from build123d import *

# Parameters (mm, degrees)
SKETCH2_R          = 1.905
CUT_EXTRUDE1_DEPTH = 2.54


with BuildPart() as part:
    # Sketch1 → Revolve1 (revolve)
    with BuildSketch(Plane.XY, mode=Mode.PRIVATE) as revolve1_sk:
        with BuildLine():
            Line((0, 0), (0.79375, 0))
            Line((0.79375, 0), (0.79375, 19.05))
            ThreePointArc((0.79375, 19.05), (0, 19.84375), (-0.79375, 19.05))
            Line((-0.79375, 19.05), (-0.79375, 0))
            Line((-0.79375, 0), (0, 0))
        make_face()
    revolve(revolve1_sk.sketch.rotate(Axis((0, 0, 0), (-1, 0, 0)), 90), axis=Axis((0, 0, 0), (-1, 0, 0)))

    # Sketch2 → Cut-Extrude1 (cut)
    with BuildSketch(Plane(origin=(0.79375, 0, 0), x_dir=(0, 0, -1), z_dir=(1, 0, 0))):
        with BuildLine():
            Line((-4.760272123, 13.32409501), (0, 4.036897437))
            Line((0, 4.036897437), (0, 14.472999652))
            ThreePointArc((0, 14.472999652), (-2.448477719, 14.181708244), (-4.760272123, 13.32409501))
        make_face()
        with BuildLine():
            Line((0, 14.472999652), (0, 4.036897437))
            Line((0, 4.036897437), (4.760272123, 13.32409501))
            ThreePointArc((4.760272123, 13.32409501), (2.448477719, 14.181708244), (0, 14.472999652))
        make_face()
        with BuildLine():
            ThreePointArc((11.200962399, 8.644659614), (13.764640629, 4.472402852), (14.142972367, -0.409916029))
            Line((14.142972367, -0.409916029), (3.839317613, 1.247469913))
            Line((3.839317613, 1.247469913), (11.200962399, 8.644659614))
        make_face()
        with BuildLine():
            ThreePointArc((11.682847592, -7.981401547), (8.507015752, -11.708902678), (3.980565502, -13.577437048))
            Line((3.980565502, -13.577437048), (2.372828779, -3.265918631))
            Line((2.372828779, -3.265918631), (11.682847592, -7.981401547))
        make_face()
        with BuildLine():
            ThreePointArc((-3.980565502, -13.577437048), (-8.507015752, -11.708902678), (-11.682847592, -7.981401547))
            Line((-11.682847592, -7.981401547), (-2.372828779, -3.265918631))
            Line((-2.372828779, -3.265918631), (-3.980565502, -13.577437048))
        make_face()
        with BuildLine():
            Line((-3.839317613, 1.247469913), (-11.200962399, 8.644659614))
            ThreePointArc((-11.200962399, 8.644659614), (-13.764640629, 4.472402852), (-14.142972367, -0.409916029))
            Line((-14.142972367, -0.409916029), (-3.839317613, 1.247469913))
        make_face()
        Circle(SKETCH2_R)
    extrude(amount=-CUT_EXTRUDE1_DEPTH, mode=Mode.SUBTRACT)


solid = part.part
Can you work these out from the model? Positions are in its coordinate system, mm. A direction names the side the tool comes from. Round coordinates to 2 decimals unless told otherwise and drop trailing zeros. Write each loop counter-clockwise with the first axis right and the second up, starting at its lowest first coordinate (ties: lowest second). Pieces come first, ordered by that corner, then holes. Notation, with made-up numbers: M 67.5,8.5 L 101.5,8.5 A24 cw 101.5,38.5 Z; hole C 10,-37 d4. An arc over 180 degrees is marked long. Use a Markdown table: item, result.
Item 1: I want a section at A-A (x = 0). List the corners of the cut face in (y, z) for me (1 decimal).
Found:
| item | result |
|---|---|
| outline | C 0,0 d39.7; hole M -13.6,-4 A10.4 ccw -8,-11.7 L -3.3,-2.4 Z; hole M -13.6,4 L -3.3,2.4 L -8,11.7 A10.4 ccw Z; hole C 0,0 d3.8; hole M -0.4,-14.1 A10.4 ccw 8.6,-11.2 L 1.2,-3.8 Z; hole M -0.4,14.1 L 1.2,3.8 L 8.6,11.2 A10.4 ccw Z; hole M 4,0 L 13.3,-4.8 A10.4 ccw 13.3,4.8 Z |
Item 2: I want a section at B-B (y = 5). State how many separate pieces and enclosed holes the cut face has, and give its area (3 significant figures).
Found:
| item | result |
|---|---|
| separate pieces | 4 |
| enclosed holes | 0 |
| area | 39.8 mm2 |
Item 3: We'd pull the mould along Z, two halves only. Please class faces 1 (the face through (0.794, 4, -0.3)), 2 (the face through (0.011, 8.746, 2.413)): released by +Z, released by -Z, zero draft, split by the parting line, or undercut.
Found:
| item | result |
|---|---|
| face 1 | zero draft |
| face 2 | undercut |
Item 4: If I drill on line 1 along Z through (x, y) = (-0.35, 8.5); line 2 along Y through (x, z) = (0.4, -10); line 3 along Z through (x, y) = (-0.4, -8.5), over which ranges is the centre line in solid material (lowest first)? Write a range as [from, to].
Found:
| item | result |
|---|---|
| line 1 | z = [-17.84, -11.34], [-11.06, -2.29], [2.29, 11.06], [11.34, 17.84] |
| line 2 | y = [-17.01, -10.39], [-7.13, 0.26], [7.44, 17.01] |
| line 3 | z = [-17.81, -11.4], [-3.19, 3.19], [11.4, 17.81] |
Item 5: Which directions (+Z, -Z, +X, -X, +Y, -Y) give clear straight access to the entire face, cutting with the end or side of a thin tool? Please do faces 3 (the face through (-0.794, 4, 0.3)), 4 (the face through (0.01, 8.62, -2.35)).
Found:
| item | result |
|---|---|
| face 3 | +Z, -Z, -X, +Y, -Y |
| face 4 | +X, -X |
